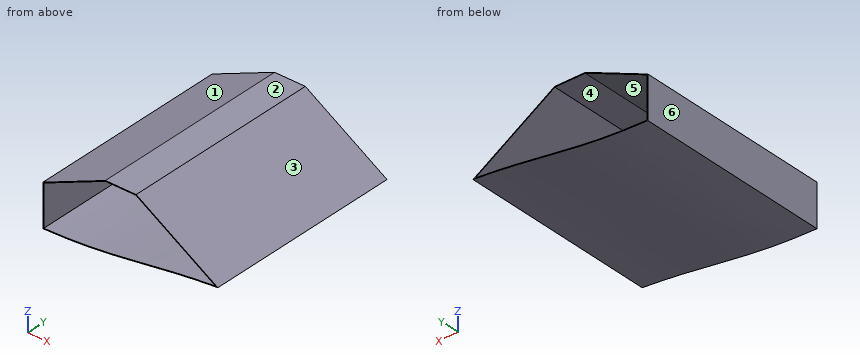
from build123d import *

# Parameters (mm, degrees)
F1_DEPTH = 528.32


# Not quite as in the source:
# - ends of sketch curves that miss each other by under 0.0002 mm in the source are joined


with BuildPart() as f1:
    # F0 (on Front) → F1 (new body)
    with BuildSketch(Plane.XZ):
        with BuildLine():
            Line((-209.5452234585, 27.1872572403), (-209.5452234585, -84.5727427597))
            add(Edge.make_bspline(
                [(-209.5452234585, -84.5727427597), (-19.6203030646, -81.5465301275), (60.0399486721, -50.63669011), (252.7347765415, -33.7727427597)],
                knots=[0, 0, 0, 0, 465.0628327441, 465.0628327441, 465.0628327441, 465.0628327441], degree=3))
            Line((252.7347765415, -33.7727427597), (36.7612242285, 99.9113052838))
            Line((36.7612242285, 99.9113052838), (-44.5187757715, 99.9113052838))
            Line((-44.5187757715, 99.9113052838), (-209.5452234585, 27.1872572403))
        make_face()
        with BuildLine():
            Line((-44.0976344097, 97.9113052838), (36.192323926, 97.9113052838))
            Line((36.192323926, 97.9113052838), (246.5747366709, -32.311920068))
            add(Edge.make_bspline(
                [(-207.545223454, -82.5394870183), (-160.9885784093, -81.7456194303), (-80.6027101112, -76.7587307387), (20.1465558538, -62.8204704396), (120.6324842882, -46.4287449505), (200.9255170344, -36.424903597), (246.5747366709, -32.311920068)],
                knots=[0.003577419, 0.003577419, 0.003577419, 0.003577419, 0.25, 0.5, 0.75, 0.9895914005, 0.9895914005, 0.9895914005, 0.9895914005], degree=3))
            Line((-207.545223454, -82.5394870183), (-207.5452234585, 25.8830305123))
            Line((-207.5452234585, 25.8830305123), (-44.0976344097, 97.9113052838))
        make_face(mode=Mode.SUBTRACT)
    extrude(amount=F1_DEPTH)


solid = f1.part
Geometry check sheet. Reference: the model listing, model coordinates, mm. Face numbers are marked on the shaded views. A direction names the side the tool comes from. Round coordinates to 2 decimals unless told otherwise and drop trailing zeros. Write each loop counter-clockwise with the first axis right and the second up, starting at its lowest first coordinate (ties: lowest second). Pieces come first, ordered by that corner, then holes. Notation, with made-up numbers: (22.25, -20.5) -> (74.25, -20.5) arc R18 ccw to (74.25, 9.5) -> close; hole circle Ø8 at (-20, -1). An arc over 180 degrees is marked (long way). One line per item, written item: value. Start each with the question number.
(1) Go/stop test with flat-tipped pins: pin 1 Ø1 at (x, y) = (-124.5, -150) entering from +Z; pin 2 Ø3 at (x, y) = (49.5, -217.5) entering from +Z; pin 3 Ø2 at (x, y) = (131.5, -108) entering from -Z. Record where each tip stops, or that it passes through.
(2) Scan lines: line 1 (Z direction, x = 219.5, y = -426); line 2 (Z direction, x = 81.5, y = -449.5); line 3 (X direction, y = -71.5, z = 18). Record each from-to range of solid material in increasing order. Write a range as [from, to].
(3) Draft check along X on the marked faces 1, 2, 3 and 4. Enter one of: +X half, -X half, draft (parallel to the pull), parting line (faces both ways), or undercut.
(4) Cross-section at B-B, the plane z = 72. Record the cut outline in (x, y), and give its area (3 significant figures).
(5) Cross-section at A-A, the plane z = -11.5. Record the cut outline in (x, y).
(6) Access from +Z, -Z, +X, -X, +Y, -Y to the whole of each face (thin tool, end or side, straight path). Record for the marked faces 5 and 6.
Answer:
1. pin 1: z = 64.89
1. pin 2: z = 92.95
1. pin 3: z = -47.75
2. line 1: [-36.92, -34.91], [-15.55, -13.2]
2. line 2: [-54.98, -52.95], [69.87, 72.22]
2. line 3: [-209.55, -207.55], [165.29, 169.09]
3. face 1: -X half
3. face 2: draft
3. face 3: +X half
3. face 4: undercut
4. outline: (-107.86, -528.32) -> (-102.9, -528.32) -> (-102.9, 0) -> (-107.86, 0) -> close; (78.05, -528.32) -> (81.85, -528.32) -> (81.85, 0) -> (78.05, 0) -> close
4. area: 4,630 mm²
5. outline: (-209.55, -528.32) -> (-207.55, -528.32) -> (-207.55, 0) -> (-209.55, 0) -> close; (212.95, -528.32) -> (216.75, -528.32) -> (216.75, 0) -> (212.95, 0) -> close
6. face 5: +Y, -Y
6. face 6: +Z, -Z, -X, +Y, -Y
